Part print with two shaded views. Sizes in mm from the minimum x, y, z corner. A direction names the side the tool comes from. Give positions to 0.01 mm unless a question says otherwise; leave off trailing zeros.
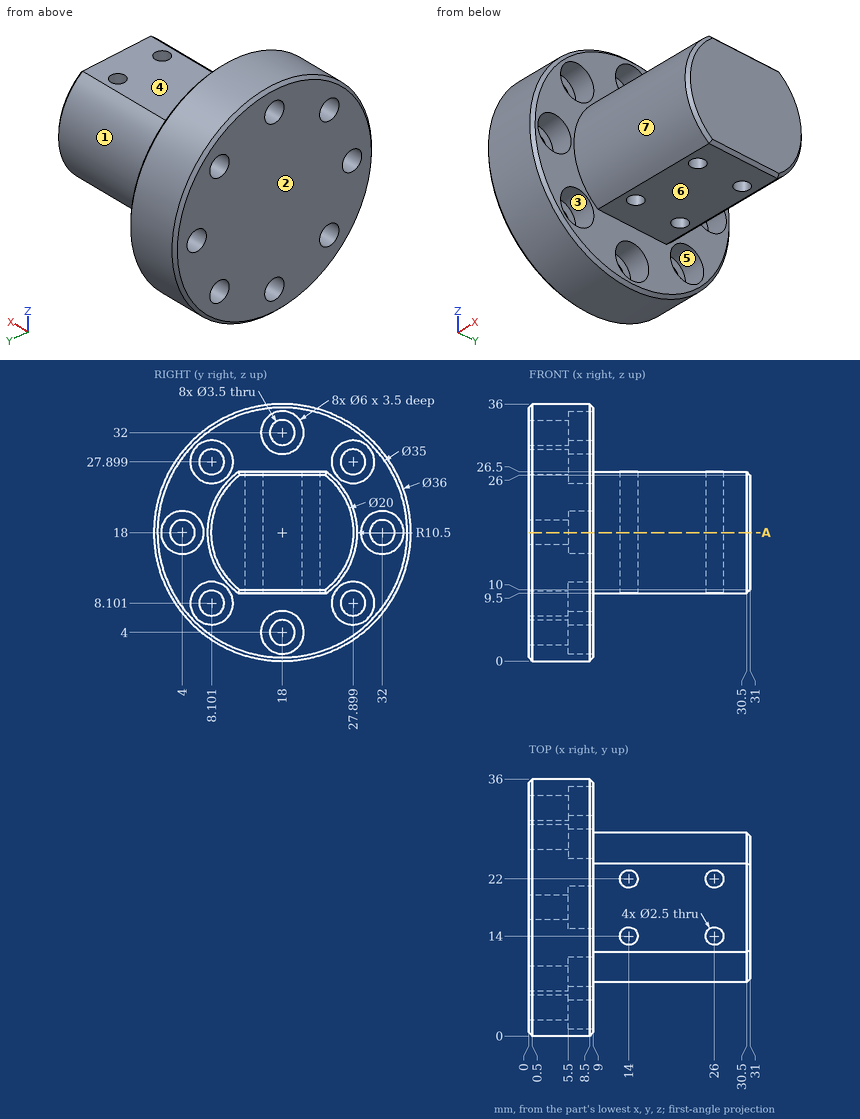
1) Saw through at A-A, the plane z = 18. Count the separate pieces of the cut face and the enclosed holes in it, then the cut area to 3 significant figures.
Answers follow:
separate pieces: 3
enclosed holes: 4
area: 685 mm2
2) Two-plate mould, pull along Z, no slides. Class the marked faces 1, 2 and 3: +Z half, -Z half, draft (parallel to the pull), parting line (faces both ways), or undercut.
Answers follow:
face 1: parting line
face 2: draft
face 3: undercut
3) 3-axis set-ups, long thin cutter, end or side, ignore diameter. For the marked faces 4, 5, 6 and 7: which of +Z, -Z, +X, -X, +Y, -Y reach the whole face in a straight line?
Answers follow:
face 4: +Z, +X, +Y, -Y
face 5: +X
face 6: -Z, +X, +Y, -Y
face 7: +X, -Y
4) Wall check: L1, parallel to X at y = 23, z = 18.5; L2, parallel to X at y = 13.5, z = 2; L3, parallel to Y at x = 27, z = 18. Give the ranges that are in metal, low to high.
Answers follow:
L1: x = 0 to 13.25, 14.75 to 25.25, 26.75 to 31
L2: x = 0 to 9
L3: y = 7.5 to 13.25, 14.75 to 21.25, 22.75 to 28.5
5) Pin check, flat tips, straight feed: pin 1 Ø1.5 at (x, z) = (10.5, 10) entering from -Y (1 decimal); pin 2 Ø5.5 at (y, z) = (18, 4) entering from -X; pin 3 Ø3 at (x, y) = (26, 14) entering from -Z; pin 4 Ø2 at (x, z) = (14, 14) entering from -Y. Stop position of each tip, or through.
Answers follow:
pin 1: stops at y = 10.4
pin 2: stops at x = 0
pin 3: stops at z = 9.5
pin 4: stops at y = 7.94
